Here's how the part is built. I have some questions about the finished solid (model axes, mm). A direction names the side the tool comes from. Round coordinates to 2 decimals unless told otherwise and drop trailing zeros. Write each loop counter-clockwise with the first axis right and the second up, starting at its lowest first coordinate (ties: lowest second). Pieces come first, ordered by that corner, then holes. Notation, with made-up numbers: (62.5, 30.5) -> (99.5, 30.5) arc R25 ccw to (99.5, 66.5) -> close; hole circle Ø2 at (-27, 56.5). An arc over 180 degrees is marked (long way). Answer as CSV lines item,"result".
```python
from build123d import *

# Parameters (mm, degrees)
SKETCH_1_R          = 6.5
EXTRUDE_1_DEPTH     = 5
SKETCH_2_R          = 7.5
EXTRUDE_2_DEPTH     = 1
SKETCH_3_R          = 3.5
CUT_EXTRUDE_1_DEPTH = 12.7260394


with BuildPart() as part:
    # ｽｹｯﾁ1 → ﾎﾞｽ - 押し出し1 (new body)
    with BuildSketch(Plane.XY):
        Circle(SKETCH_1_R)
    extrude(amount=EXTRUDE_1_DEPTH)

    # ｽｹｯﾁ2 → ﾎﾞｽ - 押し出し2 (add)
    with BuildSketch(Plane(origin=(0, 0, 0), x_dir=(-1, 0, 0), z_dir=(0, 0, -1))):
        Circle(SKETCH_2_R)
    extrude(amount=-EXTRUDE_2_DEPTH)

    # ｽｹｯﾁ3 → ｶｯﾄ - 押し出し1 (cut, through all)
    with BuildSketch(Plane.XY.offset(5)):
        Circle(SKETCH_3_R)
    extrude(amount=-CUT_EXTRUDE_1_DEPTH, mode=Mode.SUBTRACT)


solid = part.part
```
1. Suppose I cut it at D-D on y = -3.75. Please give me the cut outline in (x, z).
Numbers:
outline,"(-6.5, 0) -> (6.5, 0) -> (6.5, 1) -> (5.31, 1) -> (5.31, 5) -> (-5.31, 5) -> (-5.31, 1) -> (-6.5, 1) -> close"
2. On a 3-axis mill with a long thin cutter (end or side, diameter ignored), from which of +Z, -Z, +X, -X, +Y, -Y can I reach the whole of each face in a straight line? I mean faces 4 (the face through (-5.158, -3.955, 2.972)), 5 (the face through (3, -3, 5)). Say none if no direction works.
Numbers:
face 4,"+Z"
face 5,"+Z, +X, -X, +Y, -Y"
3. Suppose I cut it at A-A on x = 0. Please give me the cut outline in (y, z), and give its area (3 significant figures).
Numbers:
outline,"(-7.5, 0) -> (-3.5, 0) -> (-3.5, 5) -> (-6.5, 5) -> (-6.5, 1) -> (-7.5, 1) -> close; (3.5, 0) -> (7.5, 0) -> (7.5, 1) -> (6.5, 1) -> (6.5, 5) -> (3.5, 5) -> close"
area,"32.0 mm^2"
4. Suppose I cut it at C-C on z = 1.3. Please give me the cut outline in (x, y).
Numbers:
outline,"circle Ø13 at (0, 0); hole circle Ø7 at (0, 0)"
5. If we mould it in two halves opening along X, with no side actions, what happens to faces 1 (the face through (7.493, 0.33, 0.493)), 2 (the face through (3.233, -1.341, 2.535)), 3 (the face through (6, 3, 1))? For each: released by +X, released by -X, zero draft, split by the parting line, or undercut.
Numbers:
face 1,"split by the parting line"
face 2,"undercut"
face 3,"zero draft"
6. If I drill on line 1 (Y direction, x = 0, z = 2.7); line 2 (Z direction, x = -2.75, y = 6.25); line 3 (Y direction, x = -1.75, z = 2.25), over which ranges is the centre line in solid material (lowest first)?
Numbers:
line 1,"y = -6.5 to -3.5, 3.5 to 6.5"
line 2,"z = 0 to 1"
line 3,"y = -6.26 to -3.03, 3.03 to 6.26"
7. For pin 1 Ø4 at (x, y) = (0, -2.5) entering from +Z, with a flat end and sliding along its axis, tell me the tip position at first contact or that it passes through.
Numbers:
pin 1,"stops at z = 5"
